Input: dimensioned drawing with shaded views. Units: mm. Origin: part minimum x, y, z. Round coordinates to 2 decimals unless told otherwise and drop trailing zeros. Order: outer loops, then holes, each group sorted by start corner. A loop starts at its lowest first (then second) coordinate and runs counter-clockwise, first axis right, second up. Notation, with made-up numbers: M 39,-36.5 L 49,-36.5 A20 cw 49,-26.5 Z; hole C 41,-9 d4. An arc over 180 degrees is marked long. Use one line per item in the form item = value. Start each with the question number.
Q1. Section C-C (y = 3). Return the cut outline in (x, z), plus the area to 3 significant figures.
Q2. Section D-D (z = 4.85). Return the cut outline in (x, y).
Q3. Pull-direction query (X, two-part tool) for the marked faces 1, 2 and 3; classes: pulls with the +X half, pulls with the -X half, needs draft (parallel to the pull), parting line crosses it, or undercut.
Q4. Material intervals for probe 1 along X at (y, z) = (2, 3); probe 2 along X at (y, z) = (5.25, 3.9) (1 decimal); probe 3 along Z at (x, y) = (22.25, 5) (1 decimal), sorted ascending.
Q5. Section A-A (x = 22). Return the cut outline in (y, z).
Q6. Section B-B (z = 3). Return the cut outline in (x, y), plus the area to 3 significant figures.
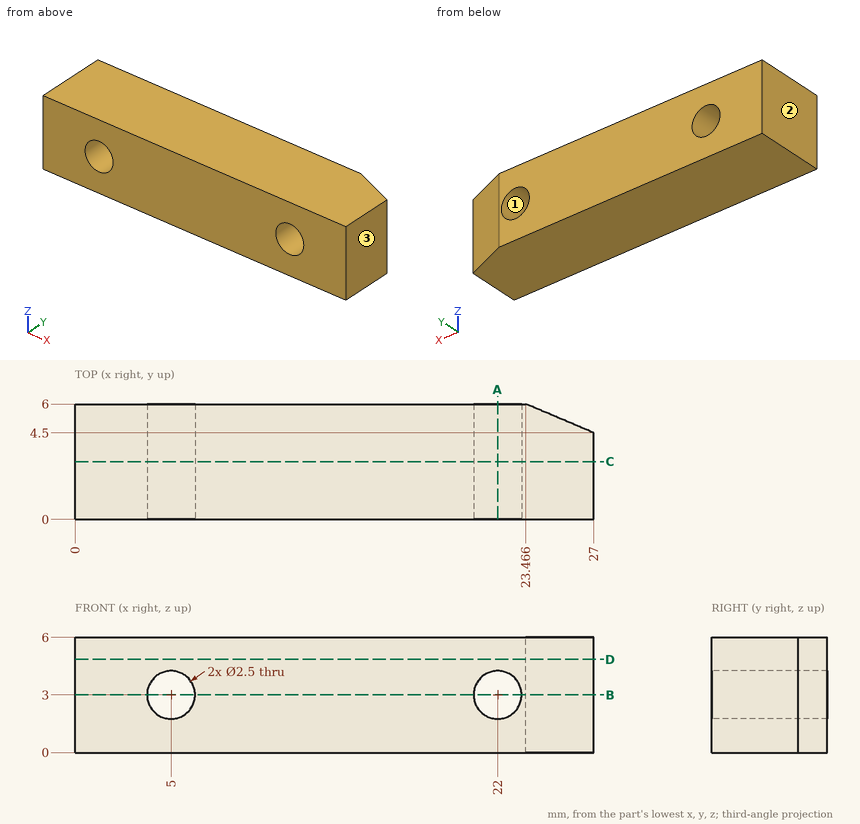
Results list:
q1.outline = M 0,0 L 27,0 L 27,6 L 0,6 Z; hole C 5,3 d2.5; hole C 22,3 d2.5
q1.area = 152 mm2
q2.outline = M 0,0 L 27,0 L 27,4.5 L 23.47,6 L 0,6 Z
q3.face_1 = undercut
q3.face_2 = pulls with the -X half
q3.face_3 = pulls with the +X half
q4.probe_1 = 0 to 3.75, 6.25 to 20.75, 23.25 to 27
q4.probe_2 = 0 to 4.1, 5.9 to 21.1, 22.9 to 25.2
q4.probe_3 = 0 to 1.8, 4.2 to 6
q5.outline = M 0,0 L 6,0 L 6,1.75 L 0,1.75 Z; M 0,4.25 L 6,4.25 L 6,6 L 0,6 Z
q6.outline = M 0,0 L 3.75,0 L 3.75,6 L 0,6 Z; M 6.25,0 L 20.75,0 L 20.75,6 L 6.25,6 Z; M 23.25,0 L 27,0 L 27,4.5 L 23.47,6 L 23.25,6 Z
q6.area = 129 mm2
